```python
from build123d import *

# Parameters (mm, degrees)
SKETCH_3_W              = 7
SKETCH_3_H              = 12
CONTINUOUS_TONGUE_DEPTH = 5
SKETCH_4_W              = 7
SKETCH_4_H              = 12
EXTRUDE_2_DEPTH         = 5
SKETCH_5_R              = 8.2
D16_CLEARANCE_DEPTH     = 25.103941586


with BuildPart() as part:
    # 草图1 → Round_nut (revolve)
    with BuildSketch(Plane.XY, mode=Mode.PRIVATE) as round_nut_sk:
        Polygon((4.2, 0), (9, 0), (9, 1), (10, 1), (10, 15), (9, 15), (9, 16), (4.2, 16), align=None)
    revolve(round_nut_sk.sketch.rotate(Axis((0, 0, 0), (0, 1, 0)), 90), axis=Axis((0, 0, 0), (0, 1, 0)))

    # 草图3 → Continuous_tongue (add)
    with BuildSketch(Plane.XY.offset(-2.5)):
        with Locations((-11.5, 8)):
            Rectangle(SKETCH_3_W, SKETCH_3_H)
    extrude(amount=CONTINUOUS_TONGUE_DEPTH)

    # 草图4 → 凸台-拉伸2 (add)
    with BuildSketch(Plane.XY.offset(-2.5)):
        with Locations((11.5, 8)):
            Rectangle(SKETCH_4_W, SKETCH_4_H)
    extrude(amount=EXTRUDE_2_DEPTH)

    # 草图5 → D16_clearance (cut, through all)
    with BuildSketch(Plane(origin=(0, 16, 0), x_dir=(1, 0, 0), z_dir=(0, 1, 0))):
        with Locations(Location((0, 0, 0), (0, 0, 270))):
            Circle(SKETCH_5_R)
    extrude(amount=-D16_CLEARANCE_DEPTH, mode=Mode.SUBTRACT)


solid = part.part
```
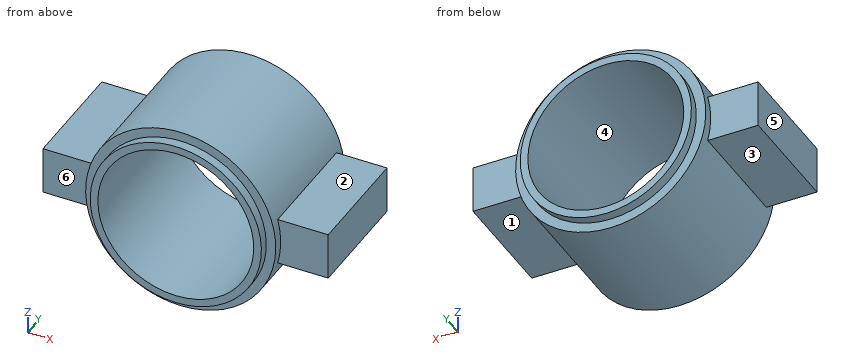
Here's how the part is built. I have some questions about the finished solid (model axes, mm). Face numbers are marked on the shaded views. A direction names the side the tool comes from. Coordinates: 2 decimals unless noted, no trailing zeros. Order: outer loops, then holes, each group sorted by start corner. A loop starts at its lowest first (then second) coordinate and runs counter-clockwise, first axis right, second up.
Item 1: If we section it at D-D, the plane z = 3: List the corners of the cut face in (x, y) for me.
Response values:
outline: (-9.54, 1) - (-8.49, 1) - (-8.49, 0) - (-7.63, 0) - (-7.63, 16) - (-8.49, 16) - (-8.49, 15) - (-9.54, 15) - close; (7.63, 0) - (8.49, 0) - (8.49, 1) - (9.54, 1) - (9.54, 15) - (8.49, 15) - (8.49, 16) - (7.63, 16) - close
Item 2: If we section it at A-A, the plane x = 0: List the corners of the cut face in (y, z) for me, then the cut area to 3 significant figures.
Response values:
outline: (0, -9) - (1, -9) - (1, -10) - (15, -10) - (15, -9) - (16, -9) - (16, -8.2) - (0, -8.2) - close; (0, 8.2) - (16, 8.2) - (16, 9) - (15, 9) - (15, 10) - (1, 10) - (1, 9) - (0, 9) - close
area: 53.6 mm2
Item 3: I'm going to push flat-ended pins straight in: pin 1 Ø5.5 at (x, z) = (12, 0.5) entering from -Y; pin 2 Ø2.5 at (x, z) = (-13.5, 0.5) entering from -Y; pin 3 Ø5 at (x, z) = (4.5, 3) entering from +Y; pin 4 Ø5.5 at (x, z) = (-12, 1) entering from +Y. Where does each tip first touch, or does it pass through?
Response values:
pin 1: stops at y = 1
pin 2: stops at y = 2
pin 3: passes through
pin 4: stops at y = 15
Item 4: Which directions (+Z, -Z, +X, -X, +Y, -Y) give clear straight access to the entire face, cutting with the end or side of a thin tool? Please do the marked faces 1, 2 and 3.
Response values:
face 1: -Z, +X, +Y, -Y
face 2: +Z, +X, +Y, -Y
face 3: -Z, -X, +Y, -Y
Item 5: I need wall thicknesses on probe 1 along X at (y, z) = (8, 0); probe 2 along X at (y, z) = (2, 4.25); probe 3 along Z at (x, y) = (3.75, 12.25). Which ranges of each line are inside material? Lowest first, please.
Response values:
probe 1: x = -15 to -8.2, 8.2 to 15
probe 2: x = -9.05 to -7.01, 7.01 to 9.05
probe 3: z = -9.27 to -7.29, 7.29 to 9.27
Item 6: If we section it at B-B, the plane z = 0: List the corners of the cut face in (x, y) for me.
Response values:
outline: (-15, 2) - (-10, 2) - (-10, 1) - (-9, 1) - (-9, 0) - (-8.2, 0) - (-8.2, 16) - (-9, 16) - (-9, 15) - (-10, 15) - (-10, 14) - (-15, 14) - close; (8.2, 0) - (9, 0) - (9, 1) - (10, 1) - (10, 2) - (15, 2) - (15, 14) - (10, 14) - (10, 15) - (9, 15) - (9, 16) - (8.2, 16) - close
Item 7: Thinking about a two-plate mould opening in X: for the marked faces 4, 5 and 6, which applies, pulls with the +X half, pulls with the -X half, needs draft (parallel to the pull), parting line crosses it, or undercut?
Response values:
face 4: undercut
face 5: pulls with the -X half
face 6: needs draft
Item 8: If we section it at C-C, the plane y = 12.5: List the corners of the cut face in (x, z) for me, then the cut area to 3 significant figures.
Response values:
outline: (-15, -2.5) - (-9.68, -2.5) arc R10 ccw to (9.68, -2.5) - (15, -2.5) - (15, 2.5) - (9.68, 2.5) arc R10 ccw to (-9.68, 2.5) - (-15, 2.5) - close; hole circle Ø16.4 at (0, 0)
area: 154 mm2
